from build123d import *

# Parameters (mm, degrees)
BOSS_EXTRUDE1_DEPTH            = 6
BOSS_EXTRUDE2_DEPTH            = 1
BOSS_EXTRUDE3_DEPTH            = 12.05
SKETCH4_R                      = 3.175
BOSS_EXTRUDE4_DEPTH            = 4
CUT_EXTRUDE1_REACH             = 87.707
SKETCH5_W                      = 14.384776311
SKETCH5_H                      = 8
CUT_EXTRUDE1_DIRECTION_2_DEPTH = 86.707273439


with BuildPart() as part:
    # Sketch1 → Boss-Extrude1 (new body)
    with BuildSketch(Plane(origin=(0, 0, 0), x_dir=(1, 0, 0), z_dir=(0, 1, 0))):
        Polygon((-54.15, 0), (-60.15, 0), (-60.15, -53.15), (-61.15, -53.15), (-61.15, -61.15), (-58.806854249, -61.15), (-31.756854249, -88.2), (0, -88.2), (0, -82.2), (-20.1, -82.2), (-20.1, -76.7), (-31.943145751, -76.7), (-38.6, -70.043145751), (-38.6, -58.2), (-53.15, -58.2), (-53.15, -53.15), (-54.15, -53.15), align=None)
    extrude(amount=BOSS_EXTRUDE1_DEPTH)

    # Sketch2 → Boss-Extrude2 (add)
    with BuildSketch(Plane.XZ):
        Polygon((-53.15, 58.2), (-53.15, 53.15), (-61.15, 53.15), (-61.15, 61.15), (-53.15, 61.15), align=None)
    extrude(amount=BOSS_EXTRUDE2_DEPTH)

    # Sketch3 → Boss-Extrude3 (add)
    with BuildSketch(Plane(origin=(0, 6, 0), x_dir=(1, 0, 0), z_dir=(0, 1, 0))):
        Polygon((-38.6, -58.2), (-44.6, -58.2), (-44.6, -72.528427125), (-34.428427125, -82.7), (-20.1, -82.7), (-20.1, -76.7), (-31.943145751, -76.7), (-38.6, -70.043145751), align=None)
    extrude(amount=BOSS_EXTRUDE3_DEPTH)

    # Sketch4 → Boss-Extrude4 (add)
    with BuildSketch(Plane(origin=(0, 18.05, 0), x_dir=(1, 0, 0), z_dir=(0, 1, 0))):
        Polygon((-44.6, -58.2), (-34.1, -58.2), (-34.1, -72.2), (-20.1, -72.2), (-20.1, -82.7), (-34.45301769, -82.7), (-40.908615626, -89.155597936), (-46.852580246, -89.155597936), (-51.055597936, -84.952580246), (-51.055597936, -79.008615626), (-44.6, -72.55301769), align=None)
        with Locations(Location((-43.880597936, -81.980597936, 0), (0, 0, 270))):
            Circle(SKETCH4_R, mode=Mode.SUBTRACT)
    extrude(amount=BOSS_EXTRUDE4_DEPTH)

    # Sketch5 → Cut-Extrude1 (cut, up to next)
    with BuildSketch(Plane(origin=(-58.564213562, 0, 58.564213562), x_dir=(0.7071067811865475, 0, 0.7071067811865477), z_dir=(-0.7071067811865477, 0, 0.7071067811865475)), mode=Mode.PRIVATE) as cut_extrude1_sk1:
        with Locations((26.940768364, 14.05)):
            Rectangle(SKETCH5_W, SKETCH5_H)
    cut_extrude1_tool1 = extrude(cut_extrude1_sk1.sketch, amount=-CUT_EXTRUDE1_REACH, mode=Mode.PRIVATE) & part.part
    add(cut_extrude1_tool1.solids().sort_by_distance((-39.514214, 14.05, 77.614214))[0], mode=Mode.SUBTRACT)

    # Sketch5 → Cut-Extrude1 direction 2 (cut)
    with BuildSketch(Plane(origin=(-58.564213562, 0, 58.564213562), x_dir=(0.7071067811865475, 0, 0.7071067811865477), z_dir=(-0.7071067811865477, 0, 0.7071067811865475))):
        with Locations((26.940768364, 14.05)):
            Rectangle(SKETCH5_W, SKETCH5_H)
    extrude(amount=CUT_EXTRUDE1_DIRECTION_2_DEPTH, mode=Mode.SUBTRACT)


solid = part.part
Input: part model. Units: mm. Frame: model coordinates. A direction names the side the tool comes from. Coordinates: 2 decimals unless noted, no trailing zeros. Loops run counter-clockwise (first coordinate to the right, second up) from the corner with the lowest first, then second, coordinate; pieces in that order, holes last.
Q1. Contact query for flat-ended pins moving along their axis: pin 1 (3.5 mm diameter, centred on y = 7, z = 64.5, fed in from +X); pin 2 (7 mm diameter, centred on x = -24, y = 13.5, fed in from +Z); pin 3 (4.5 mm diameter, centred on x = -24.5, y = 19, fed in from -Z). Output: stop coordinate, or through.
Q2. Cut plane D-D (z = 80.5). Output: boundary loops of the cut face in (x, y).
Q3. Material intervals for line 1 (Z direction, x = -24, y = 19); line 2 (X direction, y = 15, z = 66); line 3 (Z direction, x = -20.5, y = 9.5), sorted ascending.
Q4. Cut plane B-B (x = -42.5). Output: boundary loops of the cut face in (y, z), then the cut area to 3 significant figures.
Q5. Cut plane A-A (y = 16.5). Output: boundary loops of the cut face in (x, z).
Q6. Set-up query: faces 1 (the face through (-27, 20, 72.2)), 2 (the face through (-45.471, 2.958, 74.486)), 3 (the face through (-25, 9, 76.7)), 4 (the face through (-27, 14, 82.7)). Return all of +Z, -Z, +X, -X, +Y, -Y with unobstructed straight access to the full face (end or side cutting, diameter ignored); none if empty.
Q7. Cut plane C-C (y = 3.5). Output: boundary loops of the cut face in (x, z).
Q8. Draft query along Y for faces 5 (the face through (-37, 10.05, 75)), 6 (the face through (-54.15, 3, 27)), 7 (the face through (-35, 22.05, 73)), 8 (the face through (-31.47, 13.99, 79.74)). Return one class per face: +Y half, -Y half, draft (parallel to the pull), parting line (faces both ways), or undercut.
Working result:
1. pin 1: stops at x = -38.6
1. pin 2: stops at z = 82.7
1. pin 3: stops at z = 72.2
2. outline: (-51.06, 18.05) - (-46.69, 18.05) - (-46.69, 22.05) - (-51.06, 22.05) - close; (-41.07, 18.05) - (-32.23, 18.05) - (-32.23, 10.05) - (-36.63, 10.05) - (-36.63, 6) - (-39.46, 6) - (-39.46, 0) - (-20.1, 0) - (-20.1, 22.05) - (-41.07, 22.05) - close
3. line 1: z = 72.2 to 82.7
3. line 2: x = -44.6 to -38.6
3. line 3: z = 76.7 to 82.7
4. outline: (0, 58.2) - (22.05, 58.2) - (22.05, 79.12) - (18.05, 79.12) - (18.05, 70.43) - (10.05, 70.43) - (10.05, 74.63) - (6, 74.63) - (6, 77.46) - (0, 77.46) - close; (18.05, 84.84) - (22.05, 84.84) - (22.05, 89.16) - (18.05, 89.16) - close
4. area: 381 mm2
5. outline: (-44.6, 58.2) - (-38.6, 58.2) - (-38.6, 66.53) - (-44.6, 72.53) - close; (-34.43, 82.7) - (-28.43, 76.7) - (-20.1, 76.7) - (-20.1, 82.7) - close
6. face 1: -Z, +X, +Y, -Y
6. face 2: +Z, -X, -Y
6. face 3: -Z, +X, -Y
6. face 4: +Z, +X, +Y
7. outline: (-61.15, 53.15) - (-60.15, 53.15) - (-60.15, 0) - (-54.15, 0) - (-54.15, 53.15) - (-53.15, 53.15) - (-53.15, 58.2) - (-38.6, 58.2) - (-38.6, 70.04) - (-31.94, 76.7) - (-20.1, 76.7) - (-20.1, 82.2) - (0, 82.2) - (0, 88.2) - (-31.76, 88.2) - (-58.81, 61.15) - (-61.15, 61.15) - close
8. face 5: undercut
8. face 6: draft
8. face 7: +Y half
8. face 8: undercut
